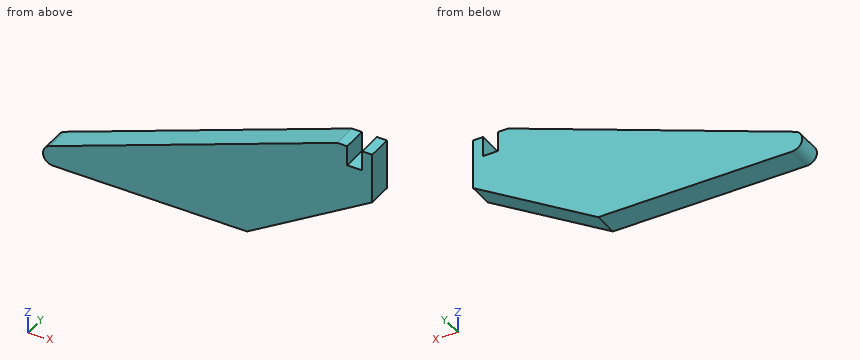
Autodesk Fusion 360 part; units mm, degrees
sketch "Sketch1" plane through (0, 0, 0) normal (0, 1, 0) x (1, 0, 0)
  line L0 (0, 0) -> (50, 0)
  line L1 (50, 0) -> (75, -15)
  line L2 (75, -15) -> (75, -25)
  line L3 (75, -25) -> (68, -25)
  line L4 (68, -25) -> (0, 0)
  line L5 (70, -25) -> (73, -25)
  line L6 (73, -25) -> (73, -21)
  line L7 (73, -21) -> (70, -21)
  line L8 (70, -21) -> (70, -25)
  dimension "d1" = 50
  dimension "d3" = 15
  dimension "d4" = 25
  dimension "d7" = 7
  dimension "d8" = 3
  dimension "d9" = 4
extrude "Extrude1" add sketch "Sketch1" along normal blind 5 contours L0 L1 L2 L3 L4 L6 L7 L8
fillet "Fillet1" radius 2 1 edges at (0, 2.5, 0)
Here's how the part is built. I have some questions about the finished solid (model axes, mm). Coordinates: 2 decimals unless noted, no trailing zeros. Write each loop counter-clockwise with the first axis right and the second up, starting at its lowest first coordinate (ties: lowest second). Pieces come first, ordered by that corner, then holes.
Item 1: I want a section at A-A on y = 2.4. Write out the boundary of the cut face in (x, z), and give its area (3 significant figures).
Item 2: Will this pin go through, and if not, where does the flat tip stop? pin 1 (1 mm diameter, centred on y = 0.5, z = 6, fed in from +X).
Item 3: I want a section at C-C on x = 27. Write out the boundary of the cut face in (y, z), and give its area (3 significant figures).
Item 4: I want a section at B-B on z = 16. Write out the boundary of the cut face in (x, y), and give its area (3 significant figures).
Item 5: If I drill on line 1 (X direction, y = 2.35, z = 2.5); line 2 (Z direction, x = 13.5, y = 0.7); line 3 (Z direction, x = 60, y = 3.9), over which ranges is the centre line in solid material (lowest first)?
Findings below:
1. outline: (10.55, 3.88) arc R2 ccw to (11.24, 0) - (50, 0) - (75, 15) - (75, 25) - (73, 25) - (73, 21) - (70, 21) - (70, 25) - (68, 25) - close
1. area: 809 mm2
2. pin 1: stops at x = 60.83
3. outline: (0, 0) - (5, 0) - (5, 9.93) - (0, 9.93) - close
3. area: 49.6 mm2
4. outline: (43.52, 0) - (75, 0) - (75, 5) - (43.52, 5) - close
4. area: 157 mm2
5. line 1: x = 9.3 to 54.17
5. line 2: z = 0 to 4.96
5. line 3: z = 6 to 22.06
